Design review of the part built by this model. Coordinates are the model's own, in mm. A direction names the side the tool comes from. Coordinates: 2 decimals unless noted, no trailing zeros. Loops run counter-clockwise (first coordinate to the right, second up) from the corner with the lowest first, then second, coordinate; pieces in that order, holes last. Notation, with made-up numbers: M -8.75,-1.75 L 30.25,-1.75 A6 ccw 30.25,2.25 Z; hole C 43,67 d3. An arc over 180 degrees is marked long. Answer as CSV lines item,"result". Start each with the question number.
from build123d import *

# Parameters (mm, degrees)
SKETCH1_W           = 240
SKETCH1_H           = 51
BOSS_EXTRUDE1_DEPTH = 5
SKETCH4_W           = 25
SKETCH4_H           = 5
BOSS_EXTRUDE2_DEPTH = 5
CUT_EXTRUDE1_DEPTH  = 10
CUT_EXTRUDE4_DEPTH  = 10
SKETCH15_W          = 25
SKETCH15_H          = 5
BOSS_EXTRUDE4_DEPTH = 5
SKETCH17_R          = 1.863928877
SKETCH17_R_2        = 1.748329033
CUT_EXTRUDE5_DEPTH  = 10
SKETCH18_R          = 4
SKETCH18_R_2        = 1.748329033
SKETCH18_R_3        = 1.863928877
BOSS_EXTRUDE5_DEPTH = 5
SKETCH19_W          = 240
SKETCH19_H          = 10
CUT_EXTRUDE6_DEPTH  = 10


with BuildPart() as part:
    # Sketch1 → Boss-Extrude1 (new body)
    with BuildSketch(Plane.XY):
        Rectangle(SKETCH1_W, SKETCH1_H)
    extrude(amount=BOSS_EXTRUDE1_DEPTH)

    # Sketch4 → Boss-Extrude2 (add)
    with BuildSketch(Plane.XY.offset(5)):
        with Locations((-69, 28)):
            Rectangle(SKETCH4_W, SKETCH4_H)
    extrude(amount=-BOSS_EXTRUDE2_DEPTH)

    # Sketch6 → Cut-Extrude1 (cut)
    with BuildSketch(Plane.XY.offset(5)):
        Polygon((-115, -4.562158061), (-120, -4.562158061), (-120, -0.562158061), (-115, -0.562158061), (-115, 0.937841939), (-111.8, 0.937841939), (-111.8, -0.562158061), (-105, -0.562158061), (-105, -4.562158061), (-111.8, -4.562158061), (-111.8, -6.062158061), (-115, -6.062158061), align=None)
    extrude(amount=-CUT_EXTRUDE1_DEPTH, mode=Mode.SUBTRACT)

    # Sketch14 → Cut-Extrude4 (cut)
    with BuildSketch(Plane.XY.offset(5)):
        with BuildLine():
            Line((-17.7, 25.5), (42.3, 25.5))
            Line((42.3, 25.5), (42.3, 3.5))
            ThreePointArc((42.3, 3.5), (39.371067812, -3.571067812), (32.3, -6.5))
            Line((32.3, -6.5), (-7.7, -6.5))
            ThreePointArc((-7.7, -6.5), (-14.771067812, -3.571067812), (-17.7, 3.5))
            Line((-17.7, 3.5), (-17.7, 25.5))
        make_face()
    extrude(amount=-CUT_EXTRUDE4_DEPTH, mode=Mode.SUBTRACT)

    # Sketch15 → Boss-Extrude4 (add)
    with BuildSketch(Plane.XY.offset(5)):
        with Locations((81.15, 28)):
            Rectangle(SKETCH15_W, SKETCH15_H)
    extrude(amount=-BOSS_EXTRUDE4_DEPTH)

    # Sketch17 → Cut-Extrude5 (cut)
    with BuildSketch(Plane.XY.offset(5)):
        with Locations((-69, 28)):
            Circle(SKETCH17_R)
        with Locations((81.151489704, 28)):
            Circle(SKETCH17_R_2)
    extrude(amount=-CUT_EXTRUDE5_DEPTH, mode=Mode.SUBTRACT)

    # Sketch18 → Boss-Extrude5 (add)
    # profile 1 of 2: a face of its own
    with BuildSketch(Plane.XY.offset(5)):
        with Locations((81.151489704, 28)):
            Circle(SKETCH18_R)
        with Locations((81.151489704, 28)):
            Circle(SKETCH18_R_2, mode=Mode.SUBTRACT)
    # profile 2 of 2: a face of its own
    with BuildSketch(Plane.XY.offset(5)):
        with Locations((-69, 28)):
            Circle(SKETCH18_R)
        with Locations((-69, 28)):
            Circle(SKETCH18_R_3, mode=Mode.SUBTRACT)
    extrude(amount=-BOSS_EXTRUDE5_DEPTH)

    # Sketch19 → Cut-Extrude6 (cut)
    with BuildSketch(Plane.XY.offset(5)):
        with Locations((0, -20.5)):
            Rectangle(SKETCH19_W, SKETCH19_H)
    extrude(amount=-CUT_EXTRUDE6_DEPTH, mode=Mode.SUBTRACT)


solid = part.part
Item 1: Mouldability with a two-part tool opening along Y and no side actions: class faces 1 (the face through (-108, -0.562, 3)), 2 (the face through (-56.5, 28, 3)), 3 (the face through (107, 25.5, 2)) as released by +Y, released by -Y, zero draft, split by the parting line, or undercut.
Item 2: For line 1 along X through (y, z) = (11, 1.7); line 2 along X through (y, z) = (29.5, 2.4); line 3 along Y through (x, z) = (-85, 4.3), list the stretches that pass through material, from the lowest coordinate up. Write a range as from..to.
Item 3: Add section C-C (x = 26). Give the boundary of the cut face in (y, z), plus the area to 3 significant figures.
Item 4: Add section A-A (y = 17). Give the boundary of the cut face in (x, z), plus the area to 3 significant figures.
Item 5: Add section B-B (z = 3.75). Give the number of separate pieces and of enclosed holes in the cut face, plus the area to 3 significant figures.
Item 6: For faces 4 (the face through (-81.5, 28, 3)), 5 (the face through (-120, -10, 2)), 6 (the face through (89, 30.5, 3)), 7 (the face through (-17.7, 14, 3)), 8 (the face through (-118, -0.562, 3)), list the 3-axis set-ups (+Z, -Z, +X, -X, +Y, -Y) from which the entire face can be reached by the end or side of a thin tool; tool diameter is ignored.
Item 7: For pin 1 (1.5 mm diameter, centred on y = 27.5, z = 2.5, fed in from +X); pin 2 (12 mm diameter, centred on x = -61, y = -5.5, fed in from -Z); pin 3 (2.5 mm diameter, centred on x = -62, z = 2.5, fed in from +Y); pin 4 (2.5 mm diameter, centred on x = 55, z = 2, fed in from +Y), all flat-tipped, find the tip position at first contact; note any pin that passes through.
Item 8: Add section D-D (x = 90.5). Give the boundary of the cut face in (y, z), plus the area to 3 significant figures.
Response:
1,face 1,"undercut"
1,face 2,"zero draft"
1,face 3,"released by +Y"
2,line 1,"-120..-17.7, 42.3..120"
2,line 2,"-81.5..-70.11, -67.89..-56.5, 68.65..80.25, 82.05..93.65"
2,line 3,"-15.5..25.5"
3,outline,"M -15.5,0 L -6.5,0 L -6.5,5 L -15.5,5 Z"
3,area,"45.0 mm²"
4,outline,"M -120,0 L -17.7,0 L -17.7,5 L -120,5 Z; M 42.3,0 L 120,0 L 120,5 L 42.3,5 Z"
4,area,"900 mm²"
5,separate pieces,"1"
5,enclosed holes,"2"
5,area,"8,140 mm²"
6,face 4,"+Z, -Z, -X, +Y"
6,face 5,"+Z, -Z, -X, +Y, -Y"
6,face 6,"+Z, -Z, +X, +Y"
6,face 7,"+Z, -Z, +Y"
6,face 8,"+Z, -Z, -X"
7,pin 1,"x = 93.65"
7,pin 2,"z = 0"
7,pin 3,"y = 30.5"
7,pin 4,"y = 25.5"
8,outline,"M -15.5,0 L 30.5,0 L 30.5,5 L -15.5,5 Z"
8,area,"230 mm²"
